```python
from build123d import *

# Parameters (mm, degrees)
CUT_EXTRUDE_1_DEPTH = 36.80502758
CHAMFER_1_SIZE      = 0.25
HOLE_WIZARD_1_D     = 4.5


# Read off the part's stored shape, not the designer's step: M4 螺纹孔1
with BuildPart() as part:
    # 草图2 → 旋转1 (revolve)
    with BuildSketch(Plane.XY, mode=Mode.PRIVATE) as revolve_1_sk:
        Polygon((32, 8), (32, 11), (12, 11), (12, 21), (6, 21), (6, 10.75), (5.5, 10.75), (5.5, 11), (0, 11), (0, 8), align=None)
    revolve(revolve_1_sk.sketch.rotate(Axis((0, 0, 0), (1, 0, 0)), 90), axis=Axis((0, 0, 0), (1, 0, 0)))

    # 草图3 → 切除-拉伸1 (cut, through all)
    with BuildSketch(Plane(origin=(12, 0, 0), x_dir=(0, 0, -1), z_dir=(1, 0, 0))):
        with BuildLine():
            Line((-13, -16.492422502), (-13, 16.492422502))
            ThreePointArc((-13, 16.492422502), (-21, 0), (-13, -16.492422502))
        make_face()
        with BuildLine():
            ThreePointArc((21, 0), (18.894443628, 9.16515139), (13, 16.492422502))
            Line((13, 16.492422502), (13, -16.492422502))
            ThreePointArc((13, -16.492422502), (18.894443628, -9.16515139), (21, 0))
        make_face()
    extrude(amount=-CUT_EXTRUDE_1_DEPTH, mode=Mode.SUBTRACT)

    # 倒角1
    chamfer_1_edges = [part.edges().sort_by_distance(p)[0] for p in [
        (0, 0, -11),
    ]]
    chamfer(chamfer_1_edges, length=CHAMFER_1_SIZE)

    # 孔1 (through all)
    with Locations(Plane(origin=(12, 0, 0), x_dir=(0, 0, -1), z_dir=(1, 0, 0))):
        with Locations((-8, 14), (-8, -14), (8, 14), (8, -14)):
            Hole(HOLE_WIZARD_1_D / 2)

    # M4 螺纹孔1 outline → M4 螺纹孔1 (revolve, cut)
    with BuildSketch(Plane(origin=(22, 0, 0), x_dir=(1, 0, 0), z_dir=(0, 0.707106781186546, 0.707106781186549))):
        Polygon((2.025041593, 11.000041593), (0, 11.000041593), (0, 7.827899387), (1.65, 7.827899387), (1.65, 10.625), align=None)
    revolve(axis=Axis((22, 0, 0), (0, 0.707106781186549, -0.707106781186546)), mode=Mode.SUBTRACT)

    # Hole Wizard M4 _1 2 outline → Hole Wizard M4 _1 2 (revolve, cut)
    with BuildSketch(Plane(origin=(22, 0, 0), x_dir=(1, 0, 0), z_dir=(0, -0.707106781186546, 0.707106781186549))):
        Polygon((0, -11.000091928), (2.025091928, -11.000091928), (1.65, -10.625), (1.65, -7.827899387), (0, -7.827899387), align=None)
    revolve(axis=Axis((22, 0, 0), (0, 0.707106781186549, 0.707106781186546)), mode=Mode.SUBTRACT)


solid = part.part
```
The listing builds one solid part. Answer for the finished solid, in the listing's coordinates (mm). A direction names the side the tool comes from. Coordinates: 2 decimals unless noted, no trailing zeros. Loops run counter-clockwise (first coordinate to the right, second up) from the corner with the lowest first, then second, coordinate; pieces in that order, holes last. Notation, with made-up numbers: (70, 32.5) -> (101, 32.5) arc R18 cw to (101, 64.5) -> close; hole circle Ø11 at (67.5, -26). An arc over 180 degrees is marked (long way). Return JSON: item names as keys, results as strings. Group by question number.
(1) A cutting plane is placed at C-C on y = 14. Write down the section's boundary in (x, z).
(2) Determine the mould class of faces 1 (the flat face through (32, 8, 2)), 2 (the cylindrical face through (9, 21, 0)), 3 (the cylindrical face through (5.75, -10.66, -1.4)) for opening direction X: released by +X, released by -X, zero draft, split by the parting line, or undercut.
(3) Given pin 1 Ø7 at (y, z) = (14, -8) entering from +X; pin 2 Ø5 at (x, z) = (22.5, 4.5) entering from +Y; pin 3 Ø6.5 at (y, z) = (-1.5, -5) entering from +X; pin 4 Ø5 at (x, y) = (25, 8.5) entering from -Z, each flat-ended and moving along its own axis, determine where each tip first touches the part or whether it passes through.
(4) A cutting plane is placed at D-D on y = 0. Write down the section's boundary in (x, z), and give its area (3 significant figures).
(5) A cutting plane is placed at B-B on z = 0. Write down the section's boundary in (x, y).
(6) Which of the six approach directions +Z, -Z, +X, -X, +Y, -Y give full straight-line access (tool end or side, diameter ignored) to faces 4 (the cylindrical face through (2.84, 10.74, -2.38)), 5 (the cylindrical face through (21.86, 4.213, 10.161)), 6 (the cylindrical face through (9, -21, 0))?
(7) Find the intervals of material crossed by probe 1 along Y at (x, z) = (20, 0); probe 2 along Z at (x, y) = (11, -15); probe 3 along Y at (x, z) = (10, 6.75), in increasing order. Write a range as from..to.
(8) A cutting plane is placed at A-A on x = 8.5. Write down the section's boundary in (y, z), and give its area (3 significant figures).
The answers:
{
 "1": {"outline": "(6, -13) -> (12, -13) -> (12, -10.25) -> (6, -10.25) -> close; (6, -5.75) -> (12, -5.75) -> (12, 5.75) -> (6, 5.75) -> close; (6, 10.25) -> (12, 10.25) -> (12, 13) -> (6, 13) -> close"},
 "2": {"face 1": "released by +X", "face 2": "zero draft", "face 3": "undercut"},
 "3": {"pin 1": "stops at x = 12", "pin 2": "stops at y = 10.82", "pin 3": "stops at x = 32", "pin 4": "stops at z = -9.22"},
 "4": {"outline": "(0, -10.75) -> (0.25, -11) -> (5.5, -11) -> (5.5, -10.75) -> (6, -10.75) -> (6, -13) -> (12, -13) -> (12, -11) -> (32, -11) -> (32, -8) -> (0, -8) -> close; (0, 8) -> (32, 8) -> (32, 11) -> (12, 11) -> (12, 13) -> (6, 13) -> (6, 10.75) -> (5.5, 10.75) -> (5.5, 11) -> (0.25, 11) -> (0, 10.75) -> close", "area": "216 mm^2"},
 "5": {"outline": "(0, -10.75) -> (0.25, -11) -> (5.5, -11) -> (5.5, -10.75) -> (6, -10.75) -> (6, -21) -> (12, -21) -> (12, -11) -> (32, -11) -> (32, -8) -> (0, -8) -> close; (0, 8) -> (32, 8) -> (32, 11) -> (12, 11) -> (12, 21) -> (6, 21) -> (6, 10.75) -> (5.5, 10.75) -> (5.5, 11) -> (0.25, 11) -> (0, 10.75) -> close"},
 "6": {"face 4": "-X", "face 5": "+X", "face 6": "+X, -X, -Y"},
 "7": {"probe 1": "y = -11..-8, 8..11", "probe 2": "z = -13..-10.02, -5.98..5.98, 10.02..13", "probe 3": "y = -19.89..-15.87, -12.13..-4.29, 4.29..12.13, 15.87..19.89"},
 "8": {"outline": "(-16.49, -13) -> (16.49, -13) arc R21 ccw to (16.49, 13) -> (-16.49, 13) arc R21 ccw to start; hole circle Ø4.5 at (-14, -8); hole circle Ø4.5 at (-14, 8); hole circle Ø16 at (0, 0); hole circle Ø4.5 at (14, -8); hole circle Ø4.5 at (14, 8)", "area": "753 mm^2"}
}
